Geometry check sheet. Reference: the model listing, model coordinates, mm. A direction names the side the tool comes from. Give positions to 0.01 mm unless a question says otherwise; leave off trailing zeros. Write each loop counter-clockwise with the first axis right and the second up, starting at its lowest first coordinate (ties: lowest second). Pieces come first, ordered by that corner, then holes. Notation, with made-up numbers: (22, -4) -> (81, -4) arc R26 ccw to (81, 20) -> close; hole circle Ø6 at (35, 78.5). An arc over 180 degrees is marked (long way). Write item = value, one per line. Start each with the question number.
1. Mould release check, pull along X, two halves, no side actions. Record for faces 1 (the conical face through (-47.1, 10.388, 32.985)), 2 (the cylindrical face through (10.27, -1.117, -25.375)), 3 (the cylindrical face through (-38.633, -7.378, -23.428)): pulls with the +X half, pulls with the -X half, needs draft (parallel to the pull), parting line crosses it, or undercut.
2. Set-up check for faces 4 (the cylindrical face through (22.473, -25.011, -20.157)), 5 (the cylindrical face through (65.301, -1.117, -25.375)), 6 (the cylindrical face through (37.57, -50.37, -6.61)): record each of +Z, -Z, +X, -X, +Y, -Y from which the full face is reachable in a straight line by a thin tool's end or side.
3. Cross-section at B-B, the plane x = 2.5. Record the cut outline in (y, z), plus the area to 3 significant figures.
4. Cross-section at C-C, the plane x = -22. Record the cut outline in (y, z).
5. Thickness scan on line 1 along Y through (x, z) = (68, 0); line 2 along Z through (x, y) = (-45.5, 8); line 3 along Z through (x, y) = (59.5, -7). Record the ranges inside material, lowest first.
6. Depth check by flat-ended pin: P1, Ø5, axis at x = -39.5, y = 6, coming from the -Z side; P2, Ø3, axis at x = -8, z = -6, coming from the -Y side; P3, Ø10, axis at x = 26.5, y = -32.5, coming from the +Z side. Enter the tip coordinate at first touch or a pass-through.
7. Cross-section at A-A, the plane z = 0. Record the cut outline in (x, y), plus the area to 3 significant figures.
```python
from build123d import *

# Parameters (mm, degrees)
SKETCH1_R           = 50.8
SKETCH1_R_2         = 25.4
BOSS_EXTRUDE1_DEPTH = 76.2
SKETCH2_R           = 50.8
BOSS_EXTRUDE2_DEPTH = 76.2
BOSS_EXTRUDE2_TAPER = 19
SKETCH3_R           = 50.8
BOSS_EXTRUDE3_DEPTH = 76.2
BOSS_EXTRUDE3_TAPER = 19
SKETCH4_R           = 24.562235867
CUT_EXTRUDE1_DEPTH  = 270.002
SKETCH5_R           = 25.4
CUT_EXTRUDE2_DEPTH  = 295.402


with BuildPart() as part:
    # Sketch1 → Boss-Extrude1 (new body)
    with BuildSketch(Plane(origin=(0, 0, 0), x_dir=(0, 0, -1), z_dir=(1, 0, 0))):
        with Locations(Location((0, 0, 0), (0, 0, 180))):
            Circle(SKETCH1_R)
        with Locations(Location((0, 0, 0), (0, 0, 180))):
            Circle(SKETCH1_R_2, mode=Mode.SUBTRACT)
    extrude(amount=BOSS_EXTRUDE1_DEPTH)

    # Sketch2 → Boss-Extrude2 (add)
    with BuildSketch(Plane.ZY):
        Circle(SKETCH2_R)
    extrude(amount=BOSS_EXTRUDE2_DEPTH, taper=BOSS_EXTRUDE2_TAPER)

    # Sketch3 → Boss-Extrude3 (add)
    with BuildSketch(Plane(origin=(76.2, 0, 0), x_dir=(0, 0, -1), z_dir=(1, 0, 0))):
        with Locations(Location((0, 0, 0), (0, 0, 180))):
            Circle(SKETCH3_R)
    extrude(amount=BOSS_EXTRUDE3_DEPTH, taper=BOSS_EXTRUDE3_TAPER)

    # Sketch4 → Cut-Extrude1 (cut)
    with BuildSketch(Plane.ZY.offset(76.2)):
        with Locations(Location((0, 0, 0), (0, 0, 180))):
            Circle(SKETCH4_R)
    extrude(amount=-CUT_EXTRUDE1_DEPTH, mode=Mode.SUBTRACT)

    # Sketch5 → Cut-Extrude2 (cut)
    with BuildSketch(Plane(origin=(0, 254, 0), x_dir=(1, 0, 0), z_dir=(0, 1, 0))):
        with Locations(Location((37.928629542, 0, 0), (0, 0, 270))):
            Circle(SKETCH5_R)
    extrude(amount=-CUT_EXTRUDE2_DEPTH, mode=Mode.SUBTRACT)


solid = part.part
```
Answers:
q1.face_1 = pulls with the -X half
q1.face_2 = undercut
q1.face_3 = needs draft
q2.face_4 = +Y
q2.face_5 = none
q2.face_6 = +X, -X
q3.outline = circle Ø101.6 at (0, 0); hole circle Ø50.8 at (0, 0)
q3.area = 6,080 mm^2
q4.outline = circle Ø86.45 at (0, 0); hole circle Ø49.12 at (0, 0)
q5.line_1 = -50.8 to -25.4, 25.4 to 50.8
q5.line_2 = -34.21 to -23.22, 23.22 to 34.21
q5.line_3 = -50.32 to -24.42, 24.42 to 50.32
q6.P1 = -37.66
q6.P2 = -48.22
q6.P3 = 42.71
q7.outline = (-76.2, -24.56) -> (0, -50.8) -> (76.2, -50.8) -> (152.4, -24.56) -> (76.2, -24.56) -> (76.2, -25.4) -> (63.33, -25.4) -> (63.33, -41.4) -> (12.53, -41.4) -> (12.53, -25.4) -> (0, -25.4) -> (0, -24.56) -> close; (-76.2, 24.56) -> (0, 24.56) -> (0, 25.4) -> (12.53, 25.4) -> (12.53, 50.8) -> (0, 50.8) -> close; (63.33, 25.4) -> (76.2, 25.4) -> (76.2, 24.56) -> (152.4, 24.56) -> (76.2, 50.8) -> (63.33, 50.8) -> close
q7.area = 5,770 mm^2
